from build123d import *

# Parameters (mm, degrees)
SKETCH1_W                     = 38
SKETCH1_H                     = 33
BOSS_EXTRUDE1_DEPTH           = 1
SKETCH2_R                     = 7.5
SKETCH2_R_2                   = 6.5
BOSS_EXTRUDE2_DEPTH           = 2
M3_CLEARANCE_HOLE1_AT_2_COUNT = 2
M3_CLEARANCE_HOLE1_AT_2_PITCH = 25
M3_CLEARANCE_HOLE1_AT_3_COUNT = 2
M3_CLEARANCE_HOLE1_AT_3_PITCH = 39.05124838
M3_CLEARANCE_HOLE1_AT_4_COUNT = 2
M3_CLEARANCE_HOLE1_AT_4_PITCH = 30
FILLET1_R                     = 2


with BuildPart() as part:
    # Sketch1 → Boss-Extrude1 (new body)
    with BuildSketch(Plane(origin=(0, 0, 0), x_dir=(1, 0, 0), z_dir=(0, 1, 0))):
        with Locations((19, 16.5)):
            Rectangle(SKETCH1_W, SKETCH1_H)
    extrude(amount=BOSS_EXTRUDE1_DEPTH)

    # Sketch2 → Boss-Extrude2 (add)
    with BuildSketch(Plane(origin=(0, 1, 0), x_dir=(1, 0, 0), z_dir=(0, 1, 0))):
        with Locations(Location((19, 16.5, 0), (0, 0, 90))):
            Circle(SKETCH2_R)
        with Locations(Location((19, 16.5, 0), (0, 0, 270))):
            Circle(SKETCH2_R_2, mode=Mode.SUBTRACT)
    extrude(amount=BOSS_EXTRUDE2_DEPTH)

    # Sketch4 → M3 Clearance Hole1 (revolve, cut)
    with BuildSketch(Plane(origin=(4, 1, -4), x_dir=(0, 0, 1), z_dir=(1, 0, 0))):
        Polygon((0, 0), (0, 1), (1.7, 1), (1.7, 0.025), (1.725, 0), align=None)
    m3_clearance_hole1 = revolve(axis=Axis((4, 7.35, -4), (0, -1, 0)), mode=Mode.SUBTRACT)

    # M3 Clearance Hole1 at 2: M3 Clearance Hole1 ×2
    with Locations(*[(0, 0, -i * M3_CLEARANCE_HOLE1_AT_2_PITCH) for i in range(1, M3_CLEARANCE_HOLE1_AT_2_COUNT)]):
        add(m3_clearance_hole1, mode=Mode.SUBTRACT)

    # M3 Clearance Hole1 at 3: M3 Clearance Hole1 ×2
    with Locations(*[Vector(0.768221279597376, 0, -0.6401843996644799) * (i * M3_CLEARANCE_HOLE1_AT_3_PITCH) for i in range(1, M3_CLEARANCE_HOLE1_AT_3_COUNT)]):
        add(m3_clearance_hole1, mode=Mode.SUBTRACT)

    # M3 Clearance Hole1 at 4: M3 Clearance Hole1 ×2
    with Locations(*[(i * M3_CLEARANCE_HOLE1_AT_4_PITCH, 0, 0) for i in range(1, M3_CLEARANCE_HOLE1_AT_4_COUNT)]):
        add(m3_clearance_hole1, mode=Mode.SUBTRACT)

    # Fillet1
    fillet1_edges = [part.edges().sort_by_distance(p)[0] for p in [
        (0, 0.5, -33),
        (38, 0.5, -33),
        (38, 0.5, 0),
        (0, 0.5, 0),
    ]]
    fillet(fillet1_edges, radius=FILLET1_R)


solid = part.part
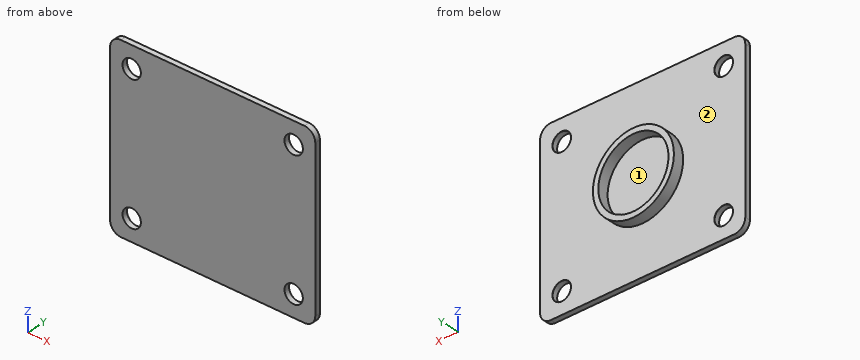
Can you work these out from the model? Positions are in its coordinate system, mm. Face numbers are marked on the shaded views. Give positions to 0.01 mm unless a question says otherwise; leave off trailing zeros. Order: outer loops, then holes, each group sorted by start corner. A loop starts at its lowest first (then second) coordinate and runs counter-clockwise, first axis right, second up. Notation, with made-up numbers: M 79.25,54 L 129.25,54 A31 ccw 129.25,79 Z; hole C 3.5,38 d3. An arc over 180 degrees is marked long. Use a Markdown table: item, result. Add a question column.
Item 1: Suppose I cut it at C-C (y = 0.5). List the corners of the cut face in (x, z) for me.
Item 2: Suppose I cut it at B-B (z = -29). List the corners of the cut face in (x, y) for me (3 decimals), then the cut area to 3 significant figures.
Item 3: If I drill on L1, parallel to X at y = 0.3, z = -4; L2, parallel to Z at x = 4, y = 0.2; L3, parallel to X at y = 2.6, z = -16.5, over which ranges is the centre line in solid material (lowest first)? Write a range as [from, to].
Item 4: Will these pins go through, and if not, where does the flat tip stop? pin 1 (1 mm diameter, centred on x = 24, z = -8, fed in from +Y); pin 2 (1 mm diameter, centred on y = 2, z = -13.5, fed in from +X).
Item 5: Suppose I cut it at D-D (x = 15). List the corners of the cut face in (y, z) for me, then the cut area to 3 significant figures.
Item 6: We'd pull the mould along Z, two halves only. Please class the marked faces 1 and 2: +Z half, -Z half, draft (parallel to the pull), parting line (faces both ways), or undercut.
Item 7: Suppose I cut it at A-A (x = 34). List the corners of the cut face in (y, z) for me (3 decimals), then the cut area to 3 significant figures.
Answer sheet:
| question | item | result |
|---|---|---|
| 1 | outline | M 0,-31 A2 ccw 2,-33 L 36,-33 A2 ccw 38,-31 L 38,-2 A2 ccw 36,0 L 2,0 A2 ccw 0,-2 Z; hole C 4,-29 d3.4; hole C 4,-4 d3.4; hole C 34,-29 d3.4; hole C 34,-4 d3.4 |
| 2 | outline | M 0,0 L 2.3,0 L 2.3,0.975 L 2.275,1 L 0,1 Z; M 5.7,0 L 32.3,0 L 32.3,0.975 L 32.275,1 L 5.725,1 L 5.7,0.975 Z; M 35.7,0 L 38,0 L 38,1 L 35.725,1 L 35.7,0.975 Z |
| 2 | area | 31.2 mm² |
| 3 | L1 | x = [0, 2.3], [5.7, 32.3], [35.7, 38] |
| 3 | L2 | z = [-33, -30.7], [-27.3, -5.7], [-2.3, 0] |
| 3 | L3 | x = [11.5, 12.5], [25.5, 26.5] |
| 4 | pin 1 | stops at y = 1 |
| 4 | pin 2 | stops at x = 26.07 |
| 5 | outline | M 0,-33 L 1,-33 L 1,-22.84 L 3,-22.84 L 3,-21.62 L 1,-21.62 L 1,-11.38 L 3,-11.38 L 3,-10.16 L 1,-10.16 L 1,0 L 0,0 Z |
| 5 | area | 37.9 mm² |
| 6 | face 1 | undercut |
| 6 | face 2 | draft |
| 7 | outline | M 0,-33 L 1,-33 L 1,-30.725 L 0.975,-30.7 L 0,-30.7 Z; M 0,-27.3 L 0.975,-27.3 L 1,-27.275 L 1,-5.725 L 0.975,-5.7 L 0,-5.7 Z; M 0,-2.3 L 0.975,-2.3 L 1,-2.275 L 1,0 L 0,0 Z |
| 7 | area | 26.2 mm² |
